from build123d import *

# Parameters (mm, degrees)
SKETCH_2_W      = 29.4
SKETCH_2_H      = 45
SKETCH_2_R      = 1.05
EXTRUDE_1_DEPTH = 1.6
SKETCH_3_W      = 13.4
SKETCH_3_H      = 5
SKETCH_3_W_2    = 15.6
EXTRUDE_2_DEPTH = 2
SKETCH_4_W      = 14.7
SKETCH_4_H      = 4
EXTRUDE_3_DEPTH = 2
SKETCH_5_W      = 8
SKETCH_5_H      = 8
EXTRUDE_4_DEPTH = 5


with BuildPart() as part:
    # 草图2 → 凸台-拉伸1 (new body)
    with BuildSketch(Plane(origin=(0, 0, 0), x_dir=(1, 0, 0), z_dir=(0, 1, 0))):
        with Locations((14.7, 22.5)):
            Rectangle(SKETCH_2_W, SKETCH_2_H)
        with Locations(Location((2, 43, 0), (0, 0, 270))):
            Circle(SKETCH_2_R, mode=Mode.SUBTRACT)
        with Locations(Location((27.4, 43, 0), (0, 0, 270))):
            Circle(SKETCH_2_R, mode=Mode.SUBTRACT)
        with Locations(Location((2, 2, 0), (0, 0, 270))):
            Circle(SKETCH_2_R, mode=Mode.SUBTRACT)
        with Locations(Location((27.4, 2, 0), (0, 0, 270))):
            Circle(SKETCH_2_R, mode=Mode.SUBTRACT)
    extrude(amount=EXTRUDE_1_DEPTH)

    # 草图3 → 凸台-拉伸2 (add)
    with BuildSketch(Plane(origin=(0, 1.6, 0), x_dir=(1, 0, 0), z_dir=(0, 1, 0))):
        with Locations((14.7, 2.5)):
            Rectangle(SKETCH_3_W, SKETCH_3_H)
        with Locations((14.7, 13.7)):
            Rectangle(SKETCH_3_W_2, SKETCH_3_H)
    extrude(amount=EXTRUDE_2_DEPTH)

    # 草图4 → 凸台-拉伸3 (add)
    with BuildSketch(Plane.XZ):
        with Locations((14.75, -4.3)):
            Rectangle(SKETCH_4_W, SKETCH_4_H)
    extrude(amount=EXTRUDE_3_DEPTH)

    # 草图5 → 凸台-拉伸4 (add)
    with BuildSketch(Plane(origin=(0, 1.6, 0), x_dir=(1, 0, 0), z_dir=(0, 1, 0))):
        with Locations((14.7, 29.6)):
            Rectangle(SKETCH_5_W, SKETCH_5_H)
    extrude(amount=EXTRUDE_4_DEPTH)


solid = part.part
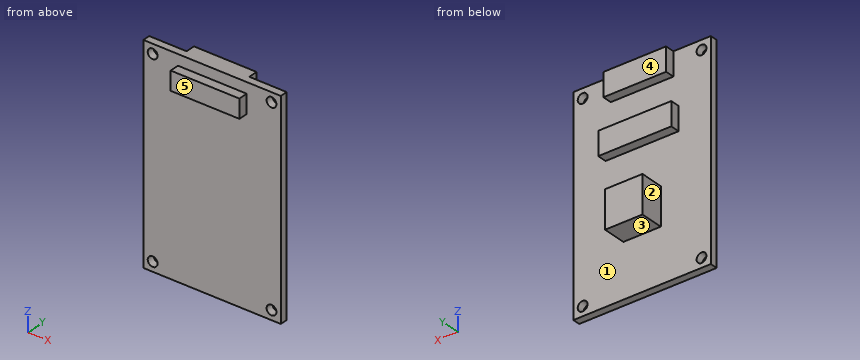
Part model, mm, in its own coordinate system. Face numbers are marked on the shaded views. A direction names the side the tool comes from. Give positions to 0.01 mm unless a question says otherwise; leave off trailing zeros. Write each loop counter-clockwise with the first axis right and the second up, starting at its lowest first coordinate (ties: lowest second). Pieces come first, ordered by that corner, then holes.
1) Which spindle directions (+Z, -Z, +X, -X, +Y, -Y) get a long thin tool onto all of the face, cutting with end or side? Do the marked faces 4 and 5. Say none if no direction does.
Resolved:
face 4: +Z, +X, -X, +Y
face 5: +Z, -Z, +X, -X, -Y
2) Cut at D-D on x = 8.5. Write the cut outline in (y, z), then the cut area to 3 significant figures.
Resolved:
outline: (-2, -6.3) - (0, -6.3) - (0, -45) - (1.6, -45) - (1.6, -16.2) - (3.6, -16.2) - (3.6, -11.2) - (1.6, -11.2) - (1.6, -5) - (3.6, -5) - (3.6, 0) - (0, 0) - (0, -2.3) - (-2, -2.3) - close
area: 100 mm2
3) Cut at A-A on y = 2.25. Write the cut outline in (x, z).
Resolved:
outline: (6.9, -16.2) - (22.5, -16.2) - (22.5, -11.2) - (6.9, -11.2) - close; (8, -5) - (21.4, -5) - (21.4, 0) - (8, 0) - close; (10.7, -33.6) - (18.7, -33.6) - (18.7, -25.6) - (10.7, -25.6) - close
4) Pin check, flat tips, straight feed: pin 1 (1 mm diameter, centred on x = 11, z = -24.5, fed in from -Y); pin 2 (1.6 mm diameter, centred on y = 3, z = -2.5, fed in from -X); pin 3 (1.6 mm diameter, centred on y = -1, z = -4.5, fed in from -X). Stop position of each tip, or through.
Resolved:
pin 1: stops at y = 0
pin 2: stops at x = 8
pin 3: stops at x = 7.4
5) Two-plate mould, pull along Z, no slides. Class the marked faces 1, 2 and 3: released by +Z, released by -Z, zero draft, split by the parting line, or undercut.
Resolved:
face 1: undercut
face 2: zero draft
face 3: released by -Z
6) Cut at B-B on x = 2. Write the cut outline in (y, z).
Resolved:
outline: (0, -45) - (1.6, -45) - (1.6, -44.05) - (0, -44.05) - close; (0, -41.95) - (1.6, -41.95) - (1.6, -3.05) - (0, -3.05) - close; (0, -0.95) - (1.6, -0.95) - (1.6, 0) - (0, 0) - close
7) Probe L1, parallel to X at y = 0.4, z = -2; L2, parallel to Y at x = 10.5, z = -36.5; L3, parallel to Z at x = 17.5, y = -0.25. List the from-to ranges inside material, lowest first.
Resolved:
L1: x = 0 to 0.95, 3.05 to 26.35, 28.45 to 29.4
L2: y = 0 to 1.6
L3: z = -6.3 to -2.3
8) Cut at C-C on z = -29. Write the cut outline in (x, y), then the cut area to 3 significant figures.
Resolved:
outline: (0, 0) - (29.4, 0) - (29.4, 1.6) - (18.7, 1.6) - (18.7, 6.6) - (10.7, 6.6) - (10.7, 1.6) - (0, 1.6) - close
area: 87.0 mm2
